Source: CAD feature listing. Evaluate the final solid. Frame: model axes, mm. A direction names the side the tool comes from. Give positions to 0.01 mm unless a question says otherwise; leave off trailing zeros. Loops run counter-clockwise (first coordinate to the right, second up) from the corner with the lowest first, then second, coordinate; pieces in that order, holes last.
from build123d import *

# Parameters (mm, degrees)
SKETCH1_R           = 4.75
BOSS_EXTRUDE1_DEPTH = 10


with BuildPart() as part:
    # Sketch1 → Boss-Extrude1 (new body)
    with BuildSketch(Plane(origin=(0, 0, 0), x_dir=(1, 0, 0), z_dir=(0, 1, 0))):
        with BuildLine():
            Line((47.257849632, 9), (-50.5, 9))
            ThreePointArc((-50.5, 9), (-59.5, 0), (-50.5, -9))
            Line((-50.5, -9), (6.281995059, -9))
            ThreePointArc((6.281995059, -9), (8.533017918, -7.587610265), (8.240583514, -4.946316871))
            ThreePointArc((8.240583514, -4.946316871), (7.841183108, 1.943198276), (14.18866595, 4.651408242))
            Line((14.18866595, 4.651408242), (36.68866595, -0.131114396))
            ThreePointArc((36.68866595, -0.131114396), (39.739895868, -1.814169405), (41.341188802, -4.909090909))
            ThreePointArc((41.341188802, -4.909090909), (43.059838886, -7.843530574), (46.257849632, -9))
            ThreePointArc((46.257849632, -9), (49.793383538, -7.535533906), (51.257849632, -4))
            Line((51.257849632, -4), (51.257849632, 5))
            ThreePointArc((51.257849632, 5), (50.086276756, 7.828427125), (47.257849632, 9))
        make_face()
        with Locations(Location((-50.5, 0, 0), (0, 0, 270))):
            Circle(SKETCH1_R, mode=Mode.SUBTRACT)
    extrude(amount=BOSS_EXTRUDE1_DEPTH)


solid = part.part
1) Contact query for a flat-ended pin moving along its axis: P1, Ø1, axis at y = 3.5, z = 6.5, coming from the +X side. Output: stop coordinate, or through.
Checks:
P1: stops at x = 50.84
2) Cut plane B-B (x = 16). Return loops of the section in (y, z), and give its area (3 significant figures).
Checks:
outline: (0, -9) - (10, -9) - (10, -4.27) - (0, -4.27) - close
area: 47.3 mm2
3) Reachability of faces 1 (the flat face through (25.281, 4.93, -2.294)), 2 (the cylindrical face through (8.516, 4.93, 7.623)), 3 (the flat face through (-5, 10, 0)) from +Z, -Z, +X, -X, +Y, -Y: full face, straight path, thin tool, end or side. Return the list, or none.
Checks:
face 1: +Z, +Y, -Y
face 2: +Y, -Y
face 3: +Z, -Z, +X, -X, +Y
4) Ray query, probe 1 along X at (y, z) = (1.5, 0.5); probe 2 along X at (y, z) = (6.75, 5.5); probe 3 along Z at (x, y) = (24, 1.5). Return the intervals inside material, ascending.
Checks:
probe 1: x = -59.49 to -55.22, -45.78 to 6.98, 37.84 to 51.26
probe 2: x = -57.62 to 8.57, 41.49 to 51.03
probe 3: z = -9 to -2.57
5) Pull-direction query (X, two-part tool) for faces 4 (the flat face through (-5, 0, 0)), 5 (the cylindrical face through (-59.498, 4.93, -0.198)), 6 (the cylindrical face through (-45.79, 4.93, -0.62)); classes: released by +X, released by -X, zero draft, split by the parting line, or undercut.
Checks:
face 4: zero draft
face 5: released by -X
face 6: undercut
6) Cut plane A-A (y = 2.25). Return loops of the section in (x, z), and give its area (3 significant figures).
Checks:
outline: (-50.5, -9) - (47.26, -9) arc R4 ccw to (51.26, -5) - (51.26, 4) arc R5 ccw to (41.34, 4.91) arc R6 cw to (36.69, 0.13) - (14.19, -4.65) arc R6 cw to (8.24, 4.95) arc R2.5 ccw to (6.28, 9) - (-50.5, 9) arc R9 ccw to start; hole circle Ø9.5 at (-50.5, 0)
area: 1,500 mm2
